Build history of the part. All positions in model axes, mm. A direction names the side the tool comes from. Coordinates: 2 decimals unless noted, no trailing zeros. Order: outer loops, then holes, each group sorted by start corner. A loop starts at its lowest first (then second) coordinate and runs counter-clockwise, first axis right, second up. Notation, with made-up numbers: (-7, 33.5) - (47, 33.5) arc R22 cw to (47, 56.5) - close; hole circle Ø8 at (-35, 35). An arc over 180 degrees is marked (long way). One line per item, written item: value.
from build123d import *

# Parameters (mm, degrees)
SKETCH1_W              = 15
SKETCH1_H              = 15
SKETCH1_W_2            = 12
SKETCH1_H_2            = 12
EXTRUDE_THIN1_DEPTH    = 221.3
CUT_EXTRUDE1_OUTLINE_R = 1.5
CUT_EXTRUDE1_DEPTH     = 15
SKETCH3_R              = 2.5
CUT_EXTRUDE2_DEPTH     = 223.314394496
SKETCH4_R              = 1.5
CUT_EXTRUDE3_DEPTH     = 223.314394496


# Read off the part's stored shape, not the designer's step: Cut-Extrude1
with BuildPart() as part:
    # Sketch1 → Extrude-Thin1 (new body)
    with BuildSketch(Plane(origin=(0, 0, 0), x_dir=(1, 0, 0), z_dir=(0, 1, 0))):
        with Locations((7.5, 7.5)):
            Rectangle(SKETCH1_W, SKETCH1_H)
        with Locations((7.5, 7.5)):
            Rectangle(SKETCH1_W_2, SKETCH1_H_2, mode=Mode.SUBTRACT)
    extrude(amount=EXTRUDE_THIN1_DEPTH)

    # Cut-Extrude1 outline → Cut-Extrude1 (cut)
    with BuildSketch(Plane.YZ):
        with Locations((12.504, -7.5)):
            Circle(CUT_EXTRUDE1_OUTLINE_R)
        with Locations((32.504, -7.5)):
            Circle(CUT_EXTRUDE1_OUTLINE_R)
        with Locations((188.8, -7.5)):
            Circle(CUT_EXTRUDE1_OUTLINE_R)
        with Locations((208.8, -7.5)):
            Circle(CUT_EXTRUDE1_OUTLINE_R)
    extrude(amount=CUT_EXTRUDE1_DEPTH, mode=Mode.SUBTRACT)

    # Sketch3 → Cut-Extrude2 (cut, through all)
    with BuildSketch(Plane(origin=(15, 0, 0), x_dir=(0, 0, -1), z_dir=(1, 0, 0))):
        with Locations((7.5, 110.65)):
            Circle(SKETCH3_R)
    extrude(amount=-CUT_EXTRUDE2_DEPTH, mode=Mode.SUBTRACT)

    # Sketch4 (on Front Plane) → Cut-Extrude3 (cut, through all)
    with BuildSketch(Plane.XY):
        with Locations((7.5, 156.8)):
            Circle(SKETCH4_R)
        with Locations((7.5, 176.8)):
            Circle(SKETCH4_R)
    extrude(amount=-CUT_EXTRUDE3_DEPTH, mode=Mode.SUBTRACT)


solid = part.part
1. Band-saw the part on A-A, the plane y = 110.65. Give the cut face in (x, z), and give its area (3 significant figures).
Values found:
outline: (0, -15) - (15, -15) - (15, -10) - (13.5, -10) - (13.5, -13.5) - (1.5, -13.5) - (1.5, -10) - (0, -10) - close; (0, -5) - (1.5, -5) - (1.5, -1.5) - (13.5, -1.5) - (13.5, -5) - (15, -5) - (15, 0) - (0, 0) - close
area: 66.0 mm2
2. Flat gauge pin, fed straight in: P1, Ø2.5, axis at x = 7.5, y = 156.8, coming from the -Z side. Where does the tip first touch, or does it go through?
Values found:
P1: passes through
3. Band-saw the part on C-C, the plane y = 83.5. Give the cut face in (x, z).
Values found:
outline: (0, -15) - (15, -15) - (15, 0) - (0, 0) - close; hole (1.5, -13.5) - (13.5, -13.5) - (13.5, -1.5) - (1.5, -1.5) - close
4. Two-plate mould, pull along X, no slides. Class faces 1 (the face through (15, 109, -4)), 2 (the face through (7, 109, -13.5)), 3 (the face through (7, 109, 0)): pulls with the +X half, pulls with the -X half, needs draft (parallel to the pull), parting line crosses it, or undercut.
Values found:
face 1: pulls with the +X half
face 2: undercut
face 3: needs draft
5. Band-saw the part on B-B, the plane x = 11.5. Give the cut face in (y, z), and give its area (3 significant figures).
Values found:
outline: (0, -15) - (221.3, -15) - (221.3, -13.5) - (0, -13.5) - close; (0, -1.5) - (221.3, -1.5) - (221.3, 0) - (0, 0) - close
area: 664 mm2
6. 3-axis set-ups, long thin cutter, end or side, ignore diameter. For faces 4 (the face through (13.5, 109, -5)), 5 (the face through (0, 109, -4)): which of +Z, -Z, +X, -X, +Y, -Y reach the whole face in a straight line?
Values found:
face 4: +Y, -Y
face 5: +Z, -Z, -X, +Y, -Y
7. Probe line 1 along Y through (x, z) = (14.15, -7.5); line 2 along X through (y, z) = (203.5, -8.5); line 3 along Z through (x, y) = (6, 209). List the from-to ranges inside material, lowest first.
Values found:
line 1: y = 0 to 11, 14 to 31, 34 to 108.15, 113.15 to 187.3, 190.3 to 207.3, 210.3 to 221.3
line 2: x = 0 to 1.5, 13.5 to 15
line 3: z = -15 to -13.5, -1.5 to 0
